The listing builds one solid part. Answer for the finished solid, in the listing's coordinates (mm). Face numbers are marked on the shaded views. A direction names the side the tool comes from. Coordinates: 2 decimals unless noted, no trailing zeros. Write each loop counter-clockwise with the first axis right and the second up, starting at its lowest first coordinate (ties: lowest second). Pieces come first, ordered by that corner, then holes.
Autodesk Inventor part; units mm, degrees
ref_plane "YZ Plane" through (0, 0, 0) normal (1, 0, 0) x (0, 1, 0)
ref_plane "XZ Plane" through (0, 0, 0) normal (0, 1, 0) x (-1, 0, 0)
ref_plane "XY Plane" through (0, 0, 0) normal (0, 0, 1) x (1, 0, 0)
sketch "Skizze1" plane through (0, 0, 0) normal (1, 0, 0) x (0, 1, 0)
  line L0 (5.5, 0) -> (32, 0)
  line L1 (32, 0) -> (32, 10.5)
  line L2 (5.5, 20) -> (5.5, 0)
  line L3 (5.5, 20) -> (20, 20)
  line L4 (20, 20) -> (20, 10.5)
  line L5 (32, 10.5) -> (20, 10.5)
  circle A0 centre (12, 15) radius 0.5
  circle A1 centre (28, 4) radius 0.5
  circle A2 centre (26, 8) radius 0.5
  line L6 (0, 24) -> (0, -4)
  line L7 (-6.4, 0) -> (38.4, 0)
  dimension "d1" = 10.5
  dimension "d3" = 20
  dimension "d21" = 1
  dimension "d28" = 1
  dimension "d31" = 4
  dimension "d41" = 1
  dimension "d43" = 8
  dimension "d54" = 5.5
  dimension "d55" = 26
  dimension "d56" = 28
  dimension "d61" = 15
  dimension "d62" = 12
  dimension "d127" = 32
  dimension "d128" = 14.5
extrude "Extrusion1" add sketch "Skizze1" along normal mid plane 6
sketch "Skizze9" plane through (-3, 0, 0) normal (-1, 0, 0) x (0, 0, 1)
  circle A0 centre (8, 26) radius 0.5
  point P0 (0, 0)
hole "Feder" at (-3, 26, 8) direction (1, 0, 0) diameter 2.459 end through all
sketch "Skizze3" plane through (-3, 0, 0) normal (-1, 0, 0) x (0, 0, 1)
  circle A0 centre (4, 28) radius 0.5
hole "Dribbler" at (-3, 28, 4) direction (1, 0, 0) diameter 4 end through all
sketch "Skizze4" plane through (-3, 0, 0) normal (-1, 0, 0) x (0, 0, 1)
  circle A0 centre (15, 12) radius 0.5
  circle A1 centre (15, 12) radius 0.5
  point P0 (0, 0)
hole "Chipper" at (-3, 12, 15) direction (1, 0, 0) diameter 4 end through all
sketch "Skizze5" plane through (3, 32, 0) normal (0, 0, -1) x (-1, 0, 0)
  line L0 (0, 0) -> (6, 0)
  line L1 (0, -26.5) -> (0, 0)
  line L2 (6, -26.5) -> (0, -26.5)
  line L3 (6, 0) -> (6, -26.5)
  line L4 (3, -26.5) -> (3, 0) construction
  point P0 (3, -10)
  point P1 (3, -24)
  point P2 (3, -17)
  point P3 (3, -13.25)
  dimension "d58" = 7
  dimension "d89" = 7
  dimension "d97" = 2.5
hole "Montage" at (0, 22, 0) at (0, 8, 0) at (0, 15, 0) direction (0, 0, 1) diameter 2.459 depth 7 tip angle 118
fillet "Rundung2" radius 2 3 edges at (0, 5.5, 20) (0, 20, 20) (0, 20, 10.5)
fillet "Rundung3" radius 4 1 edges at (0, 32, 10.5)
sketch "Skizze6" plane through (-3, 0, 0) normal (-1, 0, 0) x (0, 0, 1)
  line L0 (0, 13.7705) -> (0, 16.2295)
  line L1 (7, 16.2295) -> (7, 13.7705)
  line L2 (0, 20.7705) -> (0, 23.2295)
  line L3 (7, 23.2295) -> (7, 20.7705)
  circle A0 centre (15, 12) radius 2
  line L4 (7, 13.7705) -> (7, 23.2295) construction
  line L5 (7, 13.7705) -> (0, 13.7705) construction
  line L6 (0, 23.2295) -> (0, 13.7705) construction
  line L7 (0, 5.5) -> (0, 32) construction
  line L8 (7, 18.5) -> (0, 18.5) construction
  line L9 (15, 12) -> (15, 7) construction
  line L10 (0, 6.7705) -> (0, 9.2295)
  line L11 (7, 9.2295) -> (7, 6.7705)
  line L12 (7, 6.7705) -> (7, 16.2295) construction
  line L13 (7, 6.7705) -> (0, 6.7705) construction
  line L14 (0, 6.7705) -> (0, 16.2295) construction
  line L15 (7, 11.5) -> (0, 11.5) construction
  point P0 (0, 0)
  point P1 (3.5, 11.5)
  point P2 (3.5, 18.5)
  point P3 (7.7388, 8)
  point P4 (3.5, 11.5)
  dimension "d71" = 5
hole "Bohrung4" [suppressed]
sketch "Skizze8" plane through (-3, 0, 0) normal (-1, 0, 0) x (0, 0, 1)
  line L0 (21, 16) -> (21, 9) construction
  line L1 (-4.2, 0) -> (25.2, 0)
  line L2 (0, 38.4) -> (0, -6.4)
  point P0 (0, 0)
  dimension "d72" = 7
  dimension "d73" = 9
  dimension "d74" = 21
hole "Bohrung5" [suppressed]
sketch "Skizze10" plane through (-3, 0, 0) normal (-1, 0, 0) x (0, 0, 1)
  line L0 (0, 13.7705) -> (0, 16.2295)
  line L1 (7, 16.2295) -> (7, 13.7705)
  line L2 (0, 6.7705) -> (0, 9.2295)
  line L3 (7, 9.2295) -> (7, 6.7705)
  line L4 (-4, 0) -> (24, 0)
  line L5 (0, 38.4) -> (0, -6.4)
  point P0 (0, 0)
  point P1 (6.85, 18.5)
  dimension "d98" = 18.5
  dimension "d99" = 6.85
hole "Alternativer Anschlag" at (-3, 18.5, 6.85) direction (1, 0, 0) diameter 2.459 end through all
properties part number "Dribbler Lagerbock" material "Aluminium 6061"
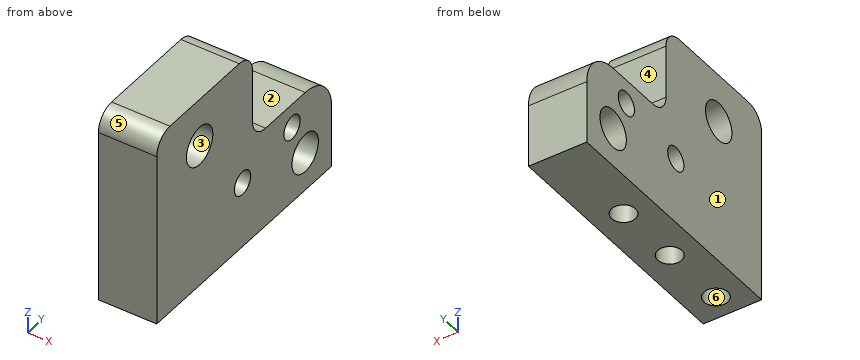
(1) Section A-A, the plane x = -1.75 is taken. Write down the section's boundary in (y, z), plus the area to 3 significant figures.
(2) Which of the six approach directions +Z, -Z, +X, -X, +Y, -Y give full straight-line access (tool end or side, diameter ignored) to the marked faces 4, 5 and 6?
(3) For a pull along Z with two mould halves and no side action, classify the marked faces 1, 2 and 3 as pulls with the +Z half, pulls with the -Z half, needs draft (parallel to the pull), parting line crosses it, or undercut.
(4) Each of these flat-tipped pins is pushed along its axis until it touches: pin 1 (2 mm diameter, centred on y = 21.5, z = 14, fed in from +X); pin 2 (3 mm diameter, centred on y = 18.5, z = 6.85, fed in from +X); pin 3 (2 mm diameter, centred on x = 0, y = 8, fed in from -Z); pin 4 (3 mm diameter, centred on x = 0, y = 26.5, fed in from +Z). Where does it stop, or does it pass through?
(5) Section B-B, the plane z = 15.25 is taken. Write down the section's boundary in (x, y).
(6) Section D-D, the plane z = 17.5 is taken. Write down the section's boundary in (x, y), plus the area to 3 significant figures.
(7) Find the intervals of material crossed by probe 1 along Z at (x, y) = (0.15, 28); probe 2 along Y at (x, z) = (1.5, 15); probe 3 along X at (y, z) = (15, 2.5), in increasing order.
(8) Section C-C, the plane y = 19 is taken. Write down the section's boundary in (x, z), plus the area to 3 significant figures.
Solution:
1. outline: (5.5, 0) - (32, 0) - (32, 6.5) arc R4 ccw to (28, 10.5) - (22, 10.5) arc R2 cw to (20, 12.5) - (20, 18) arc R2 ccw to (18, 20) - (7.5, 20) arc R2 ccw to (5.5, 18) - close; hole circle Ø4 at (12, 15); hole circle Ø2.46 at (18.5, 6.85); hole circle Ø2.46 at (26, 8); hole circle Ø4 at (28, 4)
1. area: 377 mm2
2. face 4: +Z, +X, -X, +Y
2. face 5: +Z, +X, -X, -Y
2. face 6: -Z
3. face 1: needs draft
3. face 2: pulls with the +Z half
3. face 3: undercut
4. pin 1: passes through
4. pin 2: stops at x = 3
4. pin 3: stops at z = 7.14
4. pin 4: stops at z = 10.5
5. outline: (-3, 5.5) - (3, 5.5) - (3, 10.02) - (-3, 10.02) - close; (-3, 13.98) - (3, 13.98) - (3, 20) - (-3, 20) - close
6. outline: (-3, 5.5) - (3, 5.5) - (3, 20) - (-3, 20) - close
6. area: 87.0 mm2
7. probe 1: z = 0 to 2, 6 to 10.5
7. probe 2: y = 5.5 to 10, 14 to 20
7. probe 3: x = -3 to -1.23, 1.23 to 3
8. outline: (-3, 0) - (3, 0) - (3, 5.73) - (-3, 5.73) - close; (-3, 7.97) - (3, 7.97) - (3, 19.73) - (-3, 19.73) - close
8. area: 105 mm2
